Design review of the part built by this model. Coordinates are the model's own, in mm. Face numbers are marked on the shaded views. A direction names the side the tool comes from. Round coordinates to 2 decimals unless told otherwise and drop trailing zeros. Write each loop counter-clockwise with the first axis right and the second up, starting at its lowest first coordinate (ties: lowest second). Pieces come first, ordered by that corner, then holes. Notation, with made-up numbers: M 53.25,-15 L 75.25,-15 A7 cw 75.25,-11 Z; hole C 3.5,9.5 d4. An arc over 180 degrees is marked long. One line per question, with ' | ' between items. Start each with the question number.
Item 1: Insertion check: pin 1 Ø4.5 at (x, y) = (-8, 6.5) entering from -Z. The pin has a flat end and moves straight along its axis. Give the tip position at first contact, or say it passes through.
Item 2: Draft analysis for pull direction X (two halves, no side actions). For the marked faces 1, 2 and 3, state which applies: released by +X, released by -X, zero draft, split by the parting line, or undercut.
Item 3: Machinability: for the marked faces 4 and 5, which of the approach directions +Z, -Z, +X, -X, +Y, -Y give a long, thin tool a straight path to every point of the face, cutting with its end or side? Answer none if there is none.
Item 4: Add section A-A, the plane y = 5. State the section outline as (x, z) points.
Item 5: Add section D-D, the plane z = 4.6. State the section outline as (x, y) points, and give its area (3 significant figures).
Item 6: Add section B-B, the plane z = 2. State the section outline as (x, y) points.
Item 7: For L1, parallel to Y at x = -9, z = 1.3; L2, parallel to X at y = 22, z = 0.6; L3, parallel to X at y = 5, z = 3.95, list the stretches that pass through material, from the lowest coordinate up.
Item 8: Add section C-C, the plane x = -7.25. State the section outline as (y, z) points.
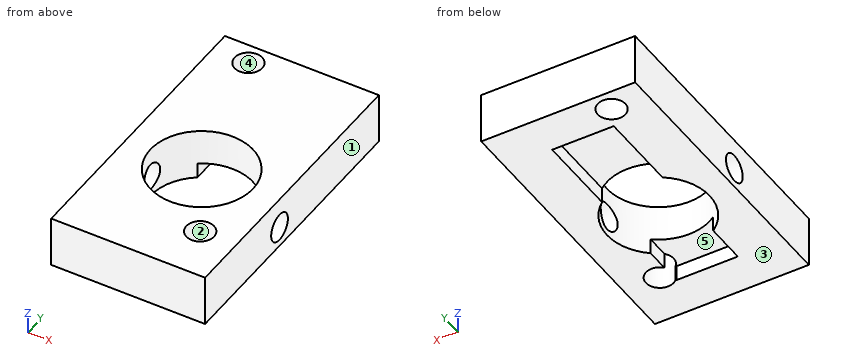
Autodesk Inventor part; units mm, degrees
ref_plane "YZ Plane" through (0, 0, 0) normal (1, 0, 0) x (0, 1, 0)
ref_plane "XZ Plane" through (0, 0, 0) normal (0, 1, 0) x (-1, 0, 0)
ref_plane "XY Plane" through (0, 0, 0) normal (0, 0, 1) x (1, 0, 0)
sketch "Sketch2" plane through (0, 0, 0) normal (0, 0, 1) x (1, 0, 0)
  line L0 (-17, 28) -> (0, 28)
  line L1 (0, 28) -> (0, 17)
  line L2 (0, 7) -> (0, 0)
  line L3 (0, 0) -> (-17, 0)
  line L4 (-17, 0) -> (-17, 7)
  line L5 (-17, 28) -> (-17, 17)
  line L6 (-17, 17) -> (-17, 7)
  line L7 (0, 17) -> (0, 7)
  dimension "d0" = 17
  dimension "d1" = 28
extrude "Extrusion1" add sketch "Sketch2" along normal blind 5
sketch "Sketch4" plane through (0, 0, 0) normal (0, 0, -1) x (-1, 0, 0)
  line L0 (17, 28) -> (0, 28)
  line L1 (0, 28) -> (0, 0)
  line L2 (0, 0) -> (17, 0)
  line L3 (17, 0) -> (17, 28)
  line L4 (0, 28) -> (17, 28)
  line L5 (11.5, 24) -> (11.5, 4)
  line L6 (11.5, 4) -> (5.5, 4)
  line L7 (5.5, 4) -> (5.5, 24)
  line L8 (5.5, 24) -> (11.5, 24)
  dimension "d15" = 6
  dimension "d17" = 5.5
  dimension "d30" = 20
  dimension "d31" = 4
extrude "Extrusion3" cut sketch "Sketch4" against normal blind 1.5 contours L5 L6 L7 L8
sketch "Sketch5" plane through (0, 0, 5) normal (0, 0, 1) x (1, 0, 0)
  line L0 (0, 28) -> (-17, 28)
  line L1 (-17, 28) -> (-17, 0)
  line L2 (-17, 0) -> (0, 0)
  line L3 (0, 0) -> (0, 28)
  line L4 (-21, 17) -> (4, 7)
  line L5 (-21.4753, 7) -> (4, 17)
  circle A0 centre (-8.6177, 12.0471) radius 5
  dimension "d20" = 10
  dimension "d21" = 12.0471
extrude "Extrusion4" cut sketch "Sketch5" against normal through all contours A0 L4 L5 | L5 L4 A0 | L4 L5 A0 | A0 L5 L4
sketch "Sketch6" plane through (0, 0, 5) normal (0, 0, 1) x (1, 0, 0)
  circle A0 centre (-8.6177, 12.0471) radius 5
  line L0 (0, 28) -> (-17, 28)
  line L1 (-17, 28) -> (-17, 0)
  line L2 (-17, 0) -> (0, 0)
  line L3 (0, 0) -> (0, 28)
  circle A1 centre (-12.5, 26) radius 1.35
  dimension "d24" = 2.7
  dimension "d25" = 4.5
  dimension "d26" = 2
extrude "Extrusion5" cut sketch "Sketch6" against normal through all contours A1
sketch "Sketch7" plane through (0, 0, 5) normal (0, 0, 1) x (1, 0, 0)
  line L0 (0, 0) -> (0, 28)
  line L1 (-17, 0) -> (0, 0)
  circle A0 centre (-4.5, 5) radius 1.35
  point P0 (0, 7)
  dimension "d32" = 2.7
  dimension "d33" = 4.5
  dimension "d34" = 5
extrude "Extrusion6" cut sketch "Sketch7" against normal through all
sketch "Sketch8" plane through (0, 0, 0) normal (1, 0, 0) x (0, 0, -1)
  circle A0 centre (-2, 12) radius 1.35
  line L0 (-5, 0) -> (-5, 28)
  line L1 (0, 0) -> (-5, 0)
  point P0 (0, -7)
  dimension "d37" = 2.7
  dimension "d41" = 12
extrude "Extrusion8" cut sketch "Sketch8" against normal through all
sketch "Sketch9" plane through (0, 0, 5) normal (0, 0, 1) x (1, 0, 0)
  circle A0 centre (-4.5, 5) radius 1.35
  circle A1 centre (-12.5, 26) radius 1.35
  circle A2 centre (-8.6177, 12.0471) radius 5
  line L0 (0, 28) -> (-17, 28)
  line L1 (-17, 28) -> (-17, 0)
  line L2 (-17, 0) -> (0, 0)
  line L3 (0, 0) -> (0, 28)
  line L4 (-17, 0) -> (-16, 0)
  line L5 (-16, 0) -> (-16, 28)
  line L6 (-16, 28) -> (-17, 28)
  line L7 (-17, 28) -> (-17, 0)
  line L8 (0, 0) -> (-1, 0)
  line L9 (-1, 0) -> (-1, 28)
  line L10 (-1, 28) -> (0, 28)
  line L11 (0, 28) -> (0, 0)
extrude "Extrusion9" cut sketch "Sketch9" against normal through all contours L3 L2 L9 L0 | L5 L2 L1 L0
properties part number "tapa0.2"
Computed values:
1) pin 1: stops at z = 1.5
2) face 1: released by +X | face 2: undercut | face 3: zero draft
3) face 4: +Z, -Z | face 5: -Z
4) outline: M -16,0 L -11.5,0 L -11.5,1.5 L -5.85,1.5 L -5.85,5 L -16,5 Z; M -3.15,0 L -1,0 L -1,5 L -3.15,5 Z
5) outline: M -16,0 L -1,0 L -1,28 L -16,28 Z; hole C -12.5,26 d2.7; hole C -8.62,12.05 d10; hole C -4.5,5 d2.7 | area: 330 mm^2
6) outline: M -16,0 L -1,0 L -1,10.65 L -3.82,10.65 A5 cw -13.42,10.65 L -16,10.65 Z; M -16,13.35 L -13.44,13.35 A5 cw -3.79,13.35 L -1,13.35 L -1,28 L -16,28 Z; hole C -12.5,26 d2.7; hole C -4.5,5 d2.7
7) L1: y = 0 to 4, 24 to 28 | L2: x = -16 to -11.5, -5.5 to -1 | L3: x = -16 to -5.85, -3.15 to -1
8) outline: M 0,0 L 4,0 L 4,1.5 L 7.24,1.5 L 7.24,5 L 0,5 Z; M 16.86,1.5 L 24,1.5 L 24,0 L 28,0 L 28,5 L 16.86,5 Z
